from build123d import *

# Parameters (mm, degrees)
CROQUIS1_R              = 100
SALIENTE_EXTRUIR1_DEPTH = 3
CROQUIS3_R              = 110
CORTAR_EXTRUIR1_DEPTH   = 3
REDONDEO1_R             = 10
CORTAR_EXTRUIR3_DEPTH   = 10
CROQUIS10_R             = 1.5
CORTAR_EXTRUIR4_DEPTH   = 142.453172607
CROQUIS11_R             = 2
CROQUIS11_W             = 17
CROQUIS11_H             = 50
CROQUIS11_W_2           = 38
CROQUIS11_H_2           = 40
CORTAR_EXTRUIR5_DEPTH   = 10
REDONDEO2_R             = 3


with BuildPart() as part:
    # Croquis1 → Saliente-Extruir1 (new body)
    with BuildSketch(Plane.XY):
        Circle(CROQUIS1_R)
    extrude(amount=SALIENTE_EXTRUIR1_DEPTH)

    # Croquis3 → Cortar-Extruir1 (cut)
    with BuildSketch(Plane.XY.offset(3)):
        with Locations((190, 0)):
            Circle(CROQUIS3_R)
    extrude(amount=-CORTAR_EXTRUIR1_DEPTH, mode=Mode.SUBTRACT)

    # Redondeo1
    redondeo1_edges = [part.edges().sort_by_distance(p)[0] for p in [
        (89.473684211, -44.659375654, 1.5),
        (89.473684211, 44.659375654, 1.5),
    ]]
    fillet(redondeo1_edges, radius=REDONDEO1_R)

    # Croquis7 → Cortar-Extruir3 (cut)
    with BuildSketch(Plane.XY.offset(3)):
        Polygon((-71.939339828, -40.119534675), (-40.119534675, -71.939339828), (-57.797204204, -89.617009358), (-89.617009358, -57.797204204), align=None)
        Polygon((-40.119534675, 71.939339828), (-71.939339828, 40.119534675), (-89.617009358, 57.797204204), (-57.797204204, 89.617009358), align=None)
        Polygon((71.939339828, 40.119534675), (40.119534675, 71.939339828), (57.797204204, 89.617009358), (89.617009358, 57.797204204), align=None)
        Polygon((40.119534675, -71.939339828), (71.939339828, -40.119534675), (89.617009358, -57.797204204), (57.797204204, -89.617009358), align=None)
    extrude(amount=-CORTAR_EXTRUIR3_DEPTH, mode=Mode.SUBTRACT)

    # Croquis10 → Cortar-Extruir4 (cut, through all)
    with BuildSketch(Plane.XY.offset(3)):
        with Locations((-20, 8.5)):
            Circle(CROQUIS10_R)
        with Locations((14.74, 72.95)):
            Circle(CROQUIS10_R)
        with Locations((-25.9, 72.95)):
            Circle(CROQUIS10_R)
        with Locations(Location((14.74, -72.95, 0), (0, 0, 180))):
            Circle(CROQUIS10_R)
        with Locations(Location((-25.9, -72.95, 0), (0, 0, 180))):
            Circle(CROQUIS10_R)
    extrude(amount=-CORTAR_EXTRUIR4_DEPTH, mode=Mode.SUBTRACT)

    # Croquis11 → Cortar-Extruir5 (cut)
    with BuildSketch(Plane.XY.offset(3)):
        with Locations((0, 92)):
            Circle(CROQUIS11_R)
        with Locations((0, -92)):
            Circle(CROQUIS11_R)
        with Locations((72, 31.694913472)):
            Circle(CROQUIS11_R)
        with Locations((72, -31.694913472)):
            Circle(CROQUIS11_R)
        with Locations((-85, -30)):
            Circle(CROQUIS11_R)
        with Locations((-85, 30)):
            Circle(CROQUIS11_R)
        with Locations((65.5, 0)):
            Rectangle(CROQUIS11_W, CROQUIS11_H)
        Polygon((55.443488939, 35.561561695), (24.824867154, 66.18018348), (13.617673752, 24.354368293), align=None)
        Polygon((13.617673752, -24.354368293), (55.443488939, -35.561561695), (24.824867154, -66.18018348), align=None)
        with Locations((-56, 0)):
            Rectangle(CROQUIS11_W_2, CROQUIS11_H_2)
    extrude(amount=-CORTAR_EXTRUIR5_DEPTH, mode=Mode.SUBTRACT)

    # Redondeo2
    redondeo2_edges = [part.edges().sort_by_distance(p)[0] for p in [
        (74, 25, 1.5),
        (74, -25, 1.5),
        (57, -25, 1.5),
        (57, 25, 1.5),
        (55.443488939, 35.561561695, 1.5),
        (13.617673752, 24.354368293, 1.5),
        (24.824867154, 66.18018348, 1.5),
        (24.824867154, -66.18018348, 1.5),
        (13.617673752, -24.354368293, 1.5),
        (55.443488939, -35.561561695, 1.5),
        (-37, 20, 1.5),
        (-37, -20, 1.5),
        (-75, -20, 1.5),
        (-75, 20, 1.5),
    ]]
    fillet(redondeo2_edges, radius=REDONDEO2_R)


solid = part.part
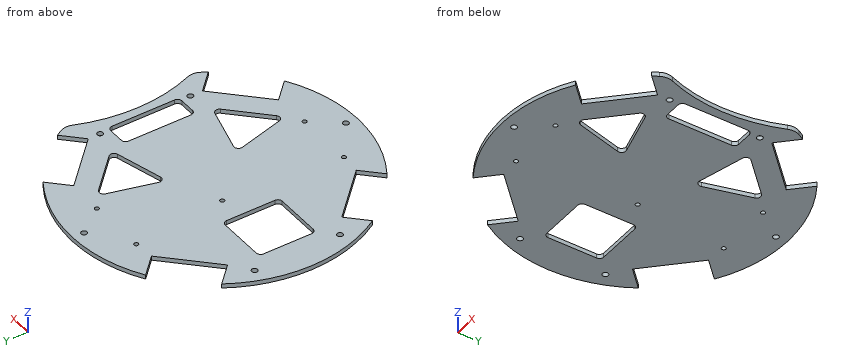
Verification items for the finished model (mm, model axes). Coordinates: 2 decimals unless noted, no trailing zeros. Write each loop counter-clockwise with the first axis right and the second up, starting at its lowest first coordinate (ties: lowest second). Pieces come first, ordered by that corner, then holes. Notation, with made-up numbers: M 28.25,81.5 L 54.25,81.5 A24 ccw 54.25,113.5 Z; hole C -10.5,13 d1. An arc over 180 degrees is marked long. Use a Markdown table: item, result.
Q1. Sectioned sample at C-C, the plane x = -31. Record the boundary of the cut face in (y, z).
Reply:
| item | result |
|---|---|
| outline | M -95.07,0 L 95.07,0 L 95.07,3 L -95.07,3 Z |
Q2. Sectioned sample at A-A, the plane y = -6.5. Record the boundary of the cut face in (x, z), plus the area to 3 significant figures.
Reply:
| item | result |
|---|---|
| outline | M -99.79,0 L -75,0 L -75,3 L -99.79,3 Z; M -37,0 L 57,0 L 57,3 L -37,3 Z; M 74,0 L 80.19,0 L 80.19,3 L 74,3 Z |
| area | 375 mm² |
Q3. Go/stop test with flat-tipped pins: P1, Ø3.5, axis at x = 14.74, y = 72.95, coming from the +Z side; P2, Ø1.5, axis at y = -10.5, z = 1, coming from the +X side; P3, Ø1.5, axis at y = 7, z = 1, coming from the +X side; P4, Ø1.5, axis at x = -53.5, z = 1.5, coming from the -Y side. Record where each tip stops, or that it passes through.
Reply:
| item | result |
|---|---|
| P1 | stops at z = 3 |
| P2 | stops at x = 80.58 |
| P3 | stops at x = 80.27 |
| P4 | stops at y = -84.96 |
Q4. Sectioned sample at D-D, the plane y = -82. Record the boundary of the cut face in (x, z), plus the area to 3 significant figures.
Reply:
| item | result |
|---|---|
| outline | M -50.18,0 L 50.18,0 L 50.18,3 L -50.18,3 Z |
| area | 301 mm² |
Q5. Thickness scan on line 1 (Y direction, x = -47, z = 2.8); line 2 (X direction, y = -46, z = 1); line 3 (Y direction, x = 72, z = 1.25). Record the ranges inside material, lowest first.
Reply:
| item | result |
|---|---|
| line 1 | y = -88.27 to -78.82, -65.06 to -20, 20 to 65.06, 78.82 to 88.27 |
| line 2 | x = -88.79 to -77.82, -66.06 to 19.42, 45.01 to 66.06, 77.82 to 88.25 |
| line 3 | y = -40.18 to -33.69, -29.69 to -24.83, 24.83 to 29.69, 33.69 to 40.18 |
Q6. Sectioned sample at B-B, the plane z = 2.5. Count the separate pieces of the cut face and the enclosed holes in it, plus the area to 3 significant figures.
Reply:
| item | result |
|---|---|
| separate pieces | 1 |
| enclosed holes | 15 |
| area | 22,600 mm² |
